Can you work these out from the model? Positions are in its coordinate system, mm. A direction names the side the tool comes from. Round coordinates to 2 decimals unless told otherwise and drop trailing zeros. Order: outer loops, then holes, each group sorted by start corner. A loop starts at its lowest first (then second) coordinate and runs counter-clockwise, first axis right, second up. Notation, with made-up numbers: (-27, 30) -> (9, 30) arc R26 cw to (9, 46) -> close; hole circle Ø11 at (64, 86). An arc over 180 degrees is marked (long way). Use a Markdown table: item, result. Add a question column.
Q1. For faces 4 (the face through (0, -14.5, 2)), 5 (the face through (-1.5, -10.56, 0.07)), which set-ups out of +Z, -Z, +X, -X, +Y, -Y let a thin tool reach every point of the face, with its end or its side?
Q2. If we section it at D-D on z = -2.5: List the corners of the cut face in (x, y) for me, plus the area to 3 significant figures.
Q3. If we section it at C-C on x = 0.85: List the corners of the cut face in (y, z) for me.
Q4. If we section it at B-B on z = 0.5: List the corners of the cut face in (x, y) for me, plus the area to 3 significant figures.
Q5. We'd pull the mould along Y, two halves only. Please class faces 1 (the face through (0, -2.7, 0)), 2 (the face through (0, -6.5, 0)), 3 (the face through (0, -4, -2.9)): +Y half, -Y half, draft (parallel to the pull), parting line (faces both ways), or undercut.
Q6. If we section it at A-A on y = -0.5: List the corners of the cut face in (x, z) for me.
Q7. I'm going to push flat-ended pins straight in: pin 1 Ø3 at (x, y) = (0, -3.5) entering from -Z; pin 2 Ø1 at (x, y) = (0.5, -1) entering from -Z; pin 3 Ø0.9 at (x, z) = (0, 0.5) entering from -Y. Where does each tip first touch, or does it pass through?
Q8. I need wall thicknesses on line 1 along Z through (x, y) = (0, -10.5); line 2 along Z through (x, y) = (-0.05, 0); line 3 along X through (y, z) = (2.5, 1). Which ranges of each line are inside material? Lowest first, please. Write a range as [from, to].
```python
from build123d import *

# Parameters (mm, degrees)
CUT_EXTRUDE_1_DEPTH = 10
EXTRUDE_2_REACH     = 8.953
SKETCH_4_W          = 5.8
SKETCH_4_H          = 2.8
SKETCH_6_W          = 5.8
SKETCH_6_H          = 2.8
EXTRUDE_4_DEPTH     = 1.95
SKETCH_7_R          = 2.9
EXTRUDE_5_DEPTH     = 9
FILLET_1_R          = 0.5
SKETCH_8_R          = 1.5
CUT_EXTRUDE_2_DEPTH = 8


with BuildPart() as part:
    # 草图1 → 旋转1 (revolve)
    with BuildSketch(Plane.XY):
        with BuildLine():
            Line((0, 4.435), (0, -4.435))
            ThreePointArc((0, -4.435), (4.435, 0), (0, 4.435))
        make_face()
    revolve(axis=Axis((0, 4.435, 0), (0, -1, 0)))

    # 草图2 → 切除-拉伸1 (cut, symmetric)
    with BuildSketch(Plane.XY):
        Polygon((-1.95, 4.9314621), (-1.95, -5.561634077), (-9.481889981, 1.10646475), align=None)
        Polygon((1.95, 4.9314621), (1.95, -5.561634077), (8.441373461, -0.109913717), align=None)
    extrude(amount=CUT_EXTRUDE_1_DEPTH, both=True, mode=Mode.SUBTRACT)

    # 草图3 → 切除-旋转1 (revolve, cut)
    with BuildSketch(Plane.ZY):
        with BuildLine():
            Line((0, 3), (0, -3))
            ThreePointArc((0, -3), (3, 0), (0, 3))
        make_face()
    revolve(axis=Axis((0, 3, 0), (0, -1, 0)), mode=Mode.SUBTRACT)

    # 凸台-拉伸2: up to this face of the body (flat: up to its plane)
    extrude_2_end = Plane(part.part.faces().sort_by_distance((-1.95, 3.870640887, 0))[0])
    # 草图4 → 凸台-拉伸2 (add, up to the picked face)
    with BuildSketch(Plane.ZY, mode=Mode.PRIVATE) as extrude_2_sk1:
        with Locations((0, -4.1)):
            Rectangle(SKETCH_4_W, SKETCH_4_H)
    extrude_2_tool1 = split(extrude(extrude_2_sk1.sketch, amount=EXTRUDE_2_REACH, mode=Mode.PRIVATE), bisect_by=extrude_2_end, keep=Keep.BOTH, mode=Mode.PRIVATE)
    add(extrude_2_tool1.solids().sort_by(Axis((0, -4.1, 0), (-1, 0, 0)))[0])

    # 草图6 → 凸台-拉伸4 (add)
    with BuildSketch(Plane(origin=(1.95, 0, 0), x_dir=(0, 0, -1), z_dir=(1, 0, 0))):
        with Locations((0, -4.1)):
            Rectangle(SKETCH_6_W, SKETCH_6_H)
    extrude(amount=-EXTRUDE_4_DEPTH)

    # 草图7 → 凸台-拉伸5 (add)
    with BuildSketch(Plane.XZ.offset(5.5)):
        with Locations(Location((0, 0, 0), (0, 0, 132.253636979))):
            Circle(SKETCH_7_R)
    extrude(amount=EXTRUDE_5_DEPTH)

    # 圆角1
    # the kernel refuses this fillet: 0.5 mm, written as the material it adds along each edge
    with BuildSketch(Plane(origin=(-1.95, -5.5, 3.396508793), x_dir=(0, 1, 0), z_dir=(0, 0, -1))) as fillet_1_piece_1_section:
        with BuildLine():
            CenterArc((FILLET_1_R, -FILLET_1_R), FILLET_1_R, 90, 90)
            Line((0, -FILLET_1_R), (0, 0))
            Line((0, 0), (FILLET_1_R, 0))
        make_face()
    fillet_1_piece_1 = extrude(amount=6.793017587, mode=Mode.PRIVATE)
    fillet_1_piece_1 = fillet_1_piece_1 & Plane(origin=(0, -5.385657526, 0), x_dir=(-0.6724137930973646, 0, 0.7401754459939985), z_dir=(0, 1, 0)) * Cylinder(2.9, 16, mode=Mode.PRIVATE)
    add(fillet_1_piece_1)
    with BuildSketch(Plane(origin=(1.95, -5.5, -3.396508793), x_dir=(0, 1, 0), z_dir=(0, 0, 1))) as fillet_1_piece_2_section:
        with BuildLine():
            CenterArc((FILLET_1_R, -FILLET_1_R), FILLET_1_R, 90, 90)
            Line((0, -FILLET_1_R), (0, 0))
            Line((0, 0), (FILLET_1_R, 0))
        make_face()
    fillet_1_piece_2 = extrude(amount=6.793017587, mode=Mode.PRIVATE)
    fillet_1_piece_2 = fillet_1_piece_2 & Plane(origin=(0, -5.385657526, 0), x_dir=(-0.6724137930973646, 0, 0.7401754459939985), z_dir=(0, 1, 0)) * Cylinder(2.9, 16, mode=Mode.PRIVATE)
    add(fillet_1_piece_2)

    # 草图8 → 切除-拉伸2 (cut)
    with BuildSketch(Plane.XZ.offset(14.5)):
        Circle(SKETCH_8_R)
    extrude(amount=-CUT_EXTRUDE_2_DEPTH, mode=Mode.SUBTRACT)


solid = part.part
```
Answer below:
| question | item | result |
|---|---|---|
| 1 | face 4 | +Z, -Z, +X, -X, -Y |
| 1 | face 5 | -Y |
| 2 | outline | (-1.95, -5.5) -> (-1.47, -5.5) -> (-1.47, -14.5) -> (1.47, -14.5) -> (1.47, -5.5) -> (1.95, -5.5) -> (1.95, 3.1) arc R3.66 ccw to (-1.95, 3.1) -> close; hole circle Ø3.32 at (0, 0) |
| 2 | area | 52.8 mm² |
| 3 | outline | (-14.5, -2.77) -> (-5.5, -2.77) -> (-5.5, -2.9) -> (-3.25, -2.9) arc R4.35 ccw (long way) to (-3.25, 2.9) -> (-5.5, 2.9) -> (-5.5, 2.77) -> (-14.5, 2.77) -> (-14.5, 1.24) -> (-6.5, 1.24) -> (-6.5, -1.24) -> (-14.5, -1.24) -> close; hole (-2.7, -0.99) arc R2.88 ccw (long way) to (-2.7, 0.99) -> close |
| 4 | outline | (-2.86, -14.5) -> (-1.41, -14.5) -> (-1.41, -6.5) -> (1.41, -6.5) -> (1.41, -14.5) -> (2.86, -14.5) -> (2.86, -5.5) -> (2.45, -5.5) arc R0.5 cw to (1.95, -5) -> (1.95, -2.22) arc R2.96 cw to (1.21, -2.7) -> (-1.21, -2.7) arc R2.96 cw to (-1.95, -2.22) -> (-1.95, -5) arc R0.5 cw to (-2.45, -5.5) -> (-2.86, -5.5) -> close; (-1.95, 2.22) arc R2.96 cw to (1.95, 2.22) -> (1.95, 3.95) arc R4.41 ccw to (-1.95, 3.95) -> close |
| 4 | area | 46.1 mm² |
| 5 | face 1 | undercut |
| 5 | face 2 | -Y half |
| 5 | face 3 | draft |
| 6 | outline | (-1.95, -3.95) arc R4.41 ccw to (1.95, -3.95) -> (1.95, -2.22) arc R2.96 cw to (-1.95, -2.22) -> close; (-1.95, 2.22) arc R2.96 cw to (1.95, 2.22) -> (1.95, 3.95) arc R4.41 ccw to (-1.95, 3.95) -> close |
| 7 | pin 1 | z = -3.96 |
| 7 | pin 2 | z = -4.39 |
| 7 | pin 3 | y = -6.5 |
| 8 | line 1 | [-2.9, -1.5], [1.5, 2.9] |
| 8 | line 2 | [-4.43, -3], [3, 4.43] |
| 8 | line 3 | [-1.95, -1.32], [1.32, 1.95] |
